Could you check a few things on this model? Use its own coordinates, in mm. A direction names the side the tool comes from. Round coordinates to 2 decimals unless told otherwise and drop trailing zeros. Loops run counter-clockwise (first coordinate to the right, second up) from the corner with the lowest first, then second, coordinate; pieces in that order, holes last.
from build123d import *

# Parameters (mm, degrees)
F0_R     = 21.35
F0_R_2   = 19.75
F1_DEPTH = 62
F3_DEPTH = 62
F4_COUNT = 12


with BuildPart() as f1:
    # F0 (on Front) → F1 (new body)
    with BuildSketch(Plane.XZ):
        Circle(F0_R)
        Circle(F0_R_2, mode=Mode.SUBTRACT)
    extrude(amount=F1_DEPTH)

    # F2 (on face) → F3 (join)
    with BuildSketch(Plane(origin=(0, 0, 0), x_dir=(-1, 0, 0), z_dir=(0, 1, 0))):
        with BuildLine():
            Line((-2.75, 22.85), (-2.75, 21.1721515203))
            ThreePointArc((-2.75, 21.1721515203), (0, 21.35), (2.75, 21.1721515203))
            Line((2.75, 21.1721515203), (2.75, 22.85))
            Line((2.75, 22.85), (1.3, 22.85))
            Line((1.3, 22.85), (1.3, 25.85))
            Line((1.3, 25.85), (-1.3, 25.85))
            Line((-1.3, 25.85), (-1.3, 22.85))
            Line((-1.3, 22.85), (-2.75, 22.85))
        make_face()
    extrude(amount=-F3_DEPTH)

    # F4: F1 ×12 about axis
    f4_axis = Axis((0, 0, 0), (0, 1, 0))


with BuildPart() as f1_1:
    add(f1.part)
    for i in range(1, F4_COUNT):
        add(f1.part.rotate(f4_axis, i * 360 / F4_COUNT))


solid = f1_1.part
Item 1: We'd pull the mould along Z, two halves only. Please class faces 4 (the flat face through (17.677, -30.566, 13.381)), 5 (the flat face through (-20.43, -30.57, 8.62)), 6 (the flat face through (-22.4, -30.6, -12.9)), 7 (the flat face through (-17.4, 0, 9.7)): released by +Z, released by -Z, zero draft, split by the parting line, or undercut.
Results list:
face 4: released by +Z
face 5: undercut
face 6: released by -Z
face 7: zero draft
Item 2: For faces 1 (the flat face through (-17.677, -30.566, -13.381)), 2 (the flat face through (20.45, -30.57, 8.63)), 3 (the flat face through (-22.85, -31, 2)), which set-ups out of +Z, -Z, +X, -X, +Y, -Y let a thin tool reach every point of the face, with its end or its side?
Results list:
face 1: -Z, +Y, -Y
face 2: +X, +Y, -Y
face 3: -X, +Y, -Y
Item 3: Will these pins go through, and if not, where does the flat tip stop? pin 1 (3 mm diameter, centred on x = -3.5, y = -34.5, fed in from +Z); pin 2 (12 mm diameter, centred on x = -7, y = -13.5, fed in from -Z); pin 3 (10 mm diameter, centred on x = 14.5, z = 2, fed in from -Y); pin 4 (3.5 mm diameter, centred on y = -39, z = 25, fed in from -X).
Results list:
pin 1: stops at z = 22.85
pin 2: stops at z = -25.85
pin 3: passes through
pin 4: stops at x = -1.3
Item 4: If we section it at A-A, the plane z = 0: Please give me the cut outline in (x, y), then the cut area to 3 significant figures.
Results list:
outline: (-25.85, -62) - (-19.75, -62) - (-19.75, 0) - (-25.85, 0) - close; (19.75, -62) - (25.85, -62) - (25.85, 0) - (19.75, 0) - close
area: 756 mm2
Item 5: If we section it at B-B, the plane x = 0: Please give me the cut outline in (y, z).
Results list:
outline: (-62, -25.85) - (0, -25.85) - (0, -19.75) - (-62, -19.75) - close; (-62, 19.75) - (0, 19.75) - (0, 25.85) - (-62, 25.85) - close
Item 6: If I drill on line 1 along X through (y, z) = (-43, 0); line 2 along X through (y, z) = (-11, 1.5), over which ranges is the centre line in solid material (lowest first)?
Results list:
line 1: x = -25.85 to -19.75, 19.75 to 25.85
line 2: x = -22.85 to -19.69, 19.69 to 22.85
